Geometry: final body of the model. Coordinates: model frame, mm. A direction names the side the tool comes from. Give positions to 0.01 mm unless a question says otherwise; leave off trailing zeros. Write each loop counter-clockwise with the first axis right and the second up, starting at its lowest first coordinate (ties: lowest second). Pieces come first, ordered by that corner, then holes. Notation, with made-up numbers: M -18.75,38 L -1.75,38 A34 cw -1.75,73 Z; hole C -20.5,54.5 d1. An arc over 180 degrees is marked long. Use one line per item in the form item = value. Start each with the question number.
Item 1: Section query B-B on x = 41. Return loops of the section in (y, z), then the cut area to 3 significant figures.
Item 2: Material intervals for line 1 along Y through (x, z) = (-32, -1); line 2 along Y through (x, z) = (4.5, 17.5); line 3 along Z through (x, y) = (-28, -20), sorted ascending. Write a range as from..to.
Item 3: Access query for faces 1 (the flat face through (-12, -31, 36.893)), 2 (the flat face through (-9, 5, 12.149)), 3 (the flat face through (20, -25.4, -34)). Directions: +Z, -Z, +X, -X, +Y, -Y. A direction counts if a zero-diameter tool reaches every point of the face in a straight line with its end or side. Return the directions, or none.
Item 4: Pull-direction query (X, two-part tool) for faces 4 (the flat face through (29.51, -12.52, -75.46)), 5 (the flat face through (-12.78, 4.72, 42.64)), 6 (the flat face through (18, -25.4, -66)), 7 (the cylindrical face through (18.99, -18.93, -14.16)); classes: released by +X, released by -X, zero draft, split by the parting line, or undercut.
Item 5: Section query C-C on y = 2. Return loops of the section in (x, z).
Item 6: Section query A-A on y = -18.5. Return loops of the section in (x, z).
Item 7: Section query D-D on z = -35.5. Return loops of the section in (x, y).
Item 8: Contact query for flat-ended pins moving along their axis: P1, Ø10, axis at x = 15, z = -68, coming from the +Y side; P2, Ø3, axis at y = 6.5, z = 20, coming from the +X side; P3, Ø1.5, axis at x = 4, y = -14, coming from the +Z side. Output: stop coordinate, or through.
from build123d import *

# Parameters (mm, degrees)
F1_DEPTH  = 25.4
F2_DEPTH  = 23.1580417603
F3_DEPTH  = 55.316273123
F4_R      = 10.5299090295
F5_DEPTH  = 108.9027523994
F7_DEPTH  = 11.9440481067
F8_R      = 6.9812840575
F9_DEPTH  = 59.2665076256
F11_DEPTH = 9.5802750438


with BuildPart() as f1:
    # F0 (on Front) → F1 (new body)
    with BuildSketch(Plane.XZ):
        Polygon((24.5958286973, 18.2494423054), (-35.2649310012, 0), (0, -84.4565883958), (59.8607596985, -66.2071460904), (0, -41.6113173931), align=None)
    extrude(amount=F1_DEPTH)

    # F2 (add): a face of the model
    f2_faces = [f1.faces().sort_by_distance(p)[0] for p in [
        (12.2979143487, -12.7, -11.6809375438),
    ]]
    extrude(f2_faces, amount=F2_DEPTH)

    # F3 (add): a face of the model
    f3_faces = [f1.faces().sort_by_distance(p)[0] for p in [
        (-5.3345511519, -12.7, 9.1247211527),
    ]]
    extrude(f3_faces, amount=F3_DEPTH)

    # F4 (on face) → F5 (cut)
    with BuildSketch(Plane(origin=(27.5947180099, 0, 8.412659926), x_dir=(0, 1, 0), z_dir=(0.956536014, 0, 0.2916142209))):
        with Locations((-11.9604282081, 37.7803184092)):
            Circle(F4_R)
    extrude(amount=-F5_DEPTH, mode=Mode.SUBTRACT)

    # F6 (on face) → F7 (join)
    with BuildSketch(Plane.XZ.offset(25.4)):
        Polygon((0, 36.8930399418), (-23.3332291245, 36.8930399418), (-24.0859165788, 12.8071308136), (0, 0), (-28.0878045399, -17.1886233206), (0, -71.279310042), (21.4203697409, -50.4126047044), (0, -28.4238799673), (33.7182840896, -20.4822248551), (24.5958286973, 18.2494423054), align=None)
    extrude(amount=F7_DEPTH)

    # F8 (on face) → F9 (cut)
    with BuildSketch(Plane.XZ.offset(37.3440481067)):
        with Locations((20.4987134784, -7.3451003991)):
            Circle(F8_R)
    extrude(amount=-F9_DEPTH, mode=Mode.SUBTRACT)

    # F10 (on face) → F11 (join)
    with BuildSketch(Plane(origin=(0, 0, 0), x_dir=(-1, 0, 0), z_dir=(0, 1, 0))):
        Polygon((16.2364837848, 12.1487083648), (16.2364837848, 41.2922068478), (9.2287091538, 44.0222509205), (2.1720913557, 41.4210605836), (2.1720913557, 12.1487083648), align=None)
    extrude(amount=F11_DEPTH)


solid = f1.part
Answer sheet:
q1.outline = M -25.4,-71.96 L 0,-71.96 L 0,-58.46 L -25.4,-58.46 Z; M -25.4,-2.76 L 0,-2.76 L 0,11.51 L -25.4,11.51 Z
q1.area = 705 mm2
q2.line_1 = -25.4..0
q2.line_2 = -37.34..0
q2.line_3 = -17.4..23.85, 38.07..60.04
q3.face_1 = +Z, +X, -X, -Y
q3.face_2 = -Z, +X, -X, +Y
q3.face_3 = +X, -Y
q4.face_4 = released by +X
q4.face_5 = released by -X
q4.face_6 = zero draft
q4.face_7 = undercut
q5.outline = M -16.24,12.15 L -2.17,12.15 L -2.17,41.42 L -9.23,44.02 L -16.24,41.29 Z
q6.outline = M -51.4,52.91 L -45.69,34.2 L 14.17,52.45 L 8.46,71.16 Z; M -40.88,18.41 L -35.26,0 L 0,-84.46 L 59.86,-66.21 L 21.42,-50.41 L 46.02,9.45 L 24.6,18.25 L 18.98,36.66 Z; hole C 20.5,-7.35 d13.96
q7.outline = M -20.44,-25.4 L -18.58,-25.4 L -18.58,-37.34 L 6.89,-37.34 L 6.89,-25.4 L 27.55,-25.4 L 27.55,0 L -20.44,0 Z
q8.P1 = 0
q8.P2 = -2.17
q8.P3 = 70.03
